from build123d import *

# Parameters (mm, degrees)
SKETCH1_W                   = 20
SKETCH1_H                   = 20
EXTRUDE1_DEPTH              = 10
SKETCH2_R                   = 6
CUT_EXTRUDE1_DEPTH          = 25.494897428
EXTRUDE2_START              = -6
SKETCH4_R                   = 6
SKETCH4_R_2                 = 3.6
EXTRUDE2_DEPTH              = 6
CUT_EXTRUDE5_DEPTH          = 1.4
SKETCH13_R                  = 3.6
EXTRUDE3_DEPTH              = 0.75
SKETCH14_W                  = 6
SKETCH14_H                  = 4.57685066
EXTRUDE4_DEPTH              = 2
EXTRUDE4_DRAFT              = 5
EXTRUDE4_PROFILE_2_DEPTH    = 2
EXTRUDE4_PROFILE_2_DRAFT    = 5
FILLET2_R                   = 2.032
CIRPATTERN1_COUNT           = 2
CIRPATTERN1_ANGLE           = 90
CIRPATTERN1_COPY_1_SKETCH_W = 6
CIRPATTERN1_COPY_1_SKETCH_H = 4.57685066
CIRPATTERN1_COPY_1_DEPTH    = 2
CIRPATTERN1_COPY_1_DRAFT    = 5
CIRPATTERN1_COPY_2_SKETCH_W = 6
CIRPATTERN1_COPY_2_SKETCH_H = 4.57685066
CIRPATTERN1_COPY_2_DEPTH    = 2
CIRPATTERN1_COPY_2_DRAFT    = 5
CIRPATTERN1_COPY_3_SKETCH_W = 6
CIRPATTERN1_COPY_3_SKETCH_H = 4.57685066
CIRPATTERN1_COPY_3_DEPTH    = 2
CIRPATTERN1_COPY_3_DRAFT    = 5
SKETCH12_W                  = 6.3
SKETCH12_H                  = 0.5
CUT_EXTRUDE6_DEPTH          = 26.476901303


with BuildPart() as part:
    # Sketch1 → Extrude1 (new, symmetric)
    with BuildSketch(Plane.XY):
        Rectangle(SKETCH1_W, SKETCH1_H)
    extrude(amount=EXTRUDE1_DEPTH, both=True)

    # Sketch2 → Cut-Extrude1 (cut, through all)
    with BuildSketch(Plane.XY.offset(10)):
        Circle(SKETCH2_R)
    cut_extrude1 = extrude(amount=-CUT_EXTRUDE1_DEPTH, mode=Mode.SUBTRACT)

    # Cut-Extrude2 cone 1 section (through the dimple's axis) → Cut-Extrude2 (revolve, cut)
    with BuildSketch(Plane(origin=(0, 0, 10), x_dir=(0, -1, 0), z_dir=(1, 0, 0))):
        Polygon((0, 0), (7.05, 0), (0, 7.05), align=None)
    cut_extrude2 = revolve(axis=Axis((0, 0, 10), (0, 0, -1)), mode=Mode.SUBTRACT)

    # Sketch4 → Extrude2 (add)
    with BuildSketch(Plane(origin=(0, 0, -10), x_dir=(-1, 0, 0), z_dir=(0, 0, -1)).offset(EXTRUDE2_START)):
        with Locations(Location((0, 0, 0), (0, 0, 180))):
            Circle(SKETCH4_R)
        Circle(SKETCH4_R_2, mode=Mode.SUBTRACT)
    extrude2 = extrude(amount=EXTRUDE2_DEPTH)

    # Sketch10 → Cut-Extrude5 (cut)
    with BuildSketch(Plane(origin=(0, 0, -10), x_dir=(-1, 0, 0), z_dir=(0, 0, -1))):
        Polygon((-5.335281374, 3.15), (-3.15, 5.335281374), (-3.15, 9.5), (3.15, 9.5), (3.15, 5.335281374), (5.335281374, 3.15), (9.5, 3.15), (9.5, -3.15), (5.335281374, -3.15), (3.15, -5.335281374), (3.15, -9.5), (-3.15, -9.5), (-3.15, -5.335281374), (-5.335281374, -3.15), (-9.5, -3.15), (-9.5, 3.15), align=None)
    cut_extrude5 = extrude(amount=-CUT_EXTRUDE5_DEPTH, mode=Mode.SUBTRACT)

    # Sketch13 → Extrude3 (add)
    with BuildSketch(Plane(origin=(0, 0, -8.6), x_dir=(-1, 0, 0), z_dir=(0, 0, -1))):
        Polygon((5.27314934, 3), (5.27314934, -3), (3, -5.27314934), (3, -9.35), (-3, -9.35), (-3, -5.27314934), (-5.27314934, -3), (-5.27314934, 3), (-3, 5.27314934), (-3, 9.35), (3, 9.35), (3, 5.27314934), align=None)
        Circle(SKETCH13_R, mode=Mode.SUBTRACT)
    extrude3 = extrude(amount=EXTRUDE3_DEPTH)


with BuildPart() as extrude4_tool:
    # Sketch14 → Extrude4 (with draft: the straight prism first)
    with BuildSketch(Plane(origin=(0, 0, -9.35), x_dir=(-1, 0, 0), z_dir=(0, 0, -1))):
        with Locations((0, 7.06157467)):
            Rectangle(SKETCH14_W, SKETCH14_H)
    extrude(amount=EXTRUDE4_DEPTH)
    # Extrude4: the draft: its side faces are tilted about the plane it starts from
    extrude4_sides = [extrude4_tool.faces().sort_by_distance(p)[0] for p in [
        (3, 7.06157467, -10.35),
        (0, 4.77314934, -10.35),
        (-3, 7.06157467, -10.35),
        (0, 9.35, -10.35),
    ]]
    draft(extrude4_sides, Plane(origin=(0, 0, -9.35), x_dir=(-1, 0, 0), z_dir=(0, 0, -1)), EXTRUDE4_DRAFT)


with BuildPart() as part_1:
    add(part.part)

    # Extrude4: add extrude4_tool
    add(extrude4_tool.part)


with BuildPart() as extrude4_profile_2_tool:
    # Sketch14 → Extrude4 profile 2 (with draft: the straight prism first)
    with BuildSketch(Plane(origin=(0, 0, -9.35), x_dir=(-1, 0, 0), z_dir=(0, 0, -1))):
        with Locations((0, -7.06157467)):
            Rectangle(SKETCH14_W, SKETCH14_H)
    extrude(amount=EXTRUDE4_PROFILE_2_DEPTH)
    # Extrude4 profile 2: the draft: its side faces are tilted about the plane it starts from
    extrude4_profile_2_sides = [extrude4_profile_2_tool.faces().sort_by_distance(p)[0] for p in [
        (0, -9.35, -10.35),
        (-3, -7.06157467, -10.35),
        (0, -4.77314934, -10.35),
        (3, -7.06157467, -10.35),
    ]]
    draft(extrude4_profile_2_sides, Plane(origin=(0, 0, -9.35), x_dir=(-1, 0, 0), z_dir=(0, 0, -1)), EXTRUDE4_PROFILE_2_DRAFT)


with BuildPart() as part_2:
    add(part_1.part)

    # Extrude4 profile 2: add extrude4_profile_2_tool
    add(extrude4_profile_2_tool.part)

    # Fillet2
    fillet2_edges = [part_2.edges().sort_by_distance(p)[0] for p in [
        (10, 0, 10),
        (-10, 0, 10),
        (0, -10, 10),
        (10, -10, 0),
        (-10, -10, 0),
    ]]
    fillet(fillet2_edges, radius=FILLET2_R)

    # Sketch9 → Revolve1 (revolve)
    with BuildSketch(Plane(origin=(0, 0, 0), x_dir=(0, 0, -1), z_dir=(1, 0, 0)), mode=Mode.PRIVATE) as revolve1_sk:
        with BuildLine():
            Line((-10, 7), (-10, 6))
            Line((-10, 6), (-7, 6))
            Line((-7, 6), (-7, 5.5))
            Line((-7, 5.5), (-10, 5.5))
            Line((-10, 5.5), (-10, 0))
            Line((-10, 0), (-11, 0))
            ThreePointArc((-11, 0), (-10.874840967, 3.508917212), (-10.5, 7))
            Line((-10.5, 7), (-10, 7))
        make_face()
    revolve1 = revolve(revolve1_sk.sketch.rotate(Axis((0, 0, 10), (0, 0, -1)), 180), axis=Axis((0, 0, 10), (0, 0, -1)))

    # CirPattern1: Cut-Extrude1, Cut-Extrude2, Extrude2, Cut-Extrude5, Extrude3, Revolve1 ×2 about axis
    cirpattern1_axis = Axis((0, 0, 0), (1, 0, 0))
    add([cut_extrude1.rotate(cirpattern1_axis, i * CIRPATTERN1_ANGLE / (CIRPATTERN1_COUNT - 1)) for i in range(1, CIRPATTERN1_COUNT)], mode=Mode.SUBTRACT)
    add([cut_extrude2.rotate(cirpattern1_axis, i * CIRPATTERN1_ANGLE / (CIRPATTERN1_COUNT - 1)) for i in range(1, CIRPATTERN1_COUNT)], mode=Mode.SUBTRACT)
    add([extrude2.rotate(cirpattern1_axis, i * CIRPATTERN1_ANGLE / (CIRPATTERN1_COUNT - 1)) for i in range(1, CIRPATTERN1_COUNT)])
    add([cut_extrude5.rotate(cirpattern1_axis, i * CIRPATTERN1_ANGLE / (CIRPATTERN1_COUNT - 1)) for i in range(1, CIRPATTERN1_COUNT)], mode=Mode.SUBTRACT)
    add([extrude3.rotate(cirpattern1_axis, i * CIRPATTERN1_ANGLE / (CIRPATTERN1_COUNT - 1)) for i in range(1, CIRPATTERN1_COUNT)])
    add([revolve1.rotate(cirpattern1_axis, i * CIRPATTERN1_ANGLE / (CIRPATTERN1_COUNT - 1)) for i in range(1, CIRPATTERN1_COUNT)])


with BuildPart() as cirpattern1_copy_1_tool:
    # CirPattern1 copy 1 sketch → CirPattern1 copy 1 (with draft: the straight prism first)
    with BuildSketch(Plane(origin=(0, 9.35, 0), x_dir=(-1, 0, 0), z_dir=(0, 1, 0))):
        with Locations((0, 7.06157467)):
            Rectangle(CIRPATTERN1_COPY_1_SKETCH_W, CIRPATTERN1_COPY_1_SKETCH_H)
    extrude(amount=CIRPATTERN1_COPY_1_DEPTH)
    # CirPattern1 copy 1: the draft: its side faces are tilted about the plane it starts from
    cirpattern1_copy_1_sides = [cirpattern1_copy_1_tool.faces().sort_by_distance(p)[0] for p in [
        (3, 10.35, 7.06157467),
        (0, 10.35, 4.77314934),
        (-3, 10.35, 7.06157467),
        (0, 10.35, 9.35),
    ]]
    draft(cirpattern1_copy_1_sides, Plane(origin=(0, 9.35, 0), x_dir=(-1, 0, 0), z_dir=(0, 1, 0)), CIRPATTERN1_COPY_1_DRAFT)


with BuildPart() as part_3:
    add(part_2.part)

    # CirPattern1 copy 1: add cirpattern1_copy_1_tool
    add(cirpattern1_copy_1_tool.part)


with BuildPart() as cirpattern1_copy_2_tool:
    # CirPattern1 copy 2 sketch → CirPattern1 copy 2 (with draft: the straight prism first)
    with BuildSketch(Plane(origin=(0, 9.35, 0), x_dir=(-1, 0, 0), z_dir=(0, 1, 0))):
        with Locations((0, -7.06157467)):
            Rectangle(CIRPATTERN1_COPY_2_SKETCH_W, CIRPATTERN1_COPY_2_SKETCH_H)
    extrude(amount=CIRPATTERN1_COPY_2_DEPTH)
    # CirPattern1 copy 2: the draft: its side faces are tilted about the plane it starts from
    cirpattern1_copy_2_sides = [cirpattern1_copy_2_tool.faces().sort_by_distance(p)[0] for p in [
        (0, 10.35, -9.35),
        (-3, 10.35, -7.06157467),
        (0, 10.35, -4.77314934),
        (3, 10.35, -7.06157467),
    ]]
    draft(cirpattern1_copy_2_sides, Plane(origin=(0, 9.35, 0), x_dir=(-1, 0, 0), z_dir=(0, 1, 0)), CIRPATTERN1_COPY_2_DRAFT)


with BuildPart() as part_4:
    add(part_3.part)

    # CirPattern1 copy 2: add cirpattern1_copy_2_tool
    add(cirpattern1_copy_2_tool.part)


with BuildPart() as cirpattern1_copy_3_tool:
    # CirPattern1 copy 3 sketch → CirPattern1 copy 3 (with draft: the straight prism first)
    with BuildSketch(Plane(origin=(0, 9.35, 0), x_dir=(-1, 0, 0), z_dir=(0, 1, 0))):
        with Locations((0, -7.06157467)):
            Rectangle(CIRPATTERN1_COPY_3_SKETCH_W, CIRPATTERN1_COPY_3_SKETCH_H)
    extrude(amount=CIRPATTERN1_COPY_3_DEPTH)
    # CirPattern1 copy 3: the draft: its side faces are tilted about the plane it starts from
    cirpattern1_copy_3_sides = [cirpattern1_copy_3_tool.faces().sort_by_distance(p)[0] for p in [
        (0, 10.35, -9.35),
        (-3, 10.35, -7.06157467),
        (0, 10.35, -4.77314934),
        (3, 10.35, -7.06157467),
    ]]
    draft(cirpattern1_copy_3_sides, Plane(origin=(0, 9.35, 0), x_dir=(-1, 0, 0), z_dir=(0, 1, 0)), CIRPATTERN1_COPY_3_DRAFT)


with BuildPart() as part_5:
    add(part_4.part)

    # CirPattern1 copy 3: add cirpattern1_copy_3_tool
    add(cirpattern1_copy_3_tool.part)

    # Sketch12 → Cut-Extrude6 (cut, through all)
    with BuildSketch(Plane.XZ.offset(-9.5)):
        with Locations((0, -9.75)):
            Rectangle(SKETCH12_W, SKETCH12_H)
    extrude(amount=-CUT_EXTRUDE6_DEPTH, mode=Mode.SUBTRACT)


solid = part_5.part
Work out the finished part from the listing and answer in its coordinate system (mm). A direction names the side the tool comes from. Give positions to 0.01 mm unless a question says otherwise; leave off trailing zeros. Answer as a JSON object with one key per item and string values. Group by question number.
1. A tool of negligible diameter and unlimited length cuts with its end or side. For faces 5 (the flat face through (-2, -10, -7)), 6 (the cylindrical face through (-3.434, 6.638, 1.081)), 7 (the flat face through (7, 3.15, -9)), from which of +Z, -Z, +X, -X, +Y, -Y can it reach the whole face along a straight path? Write none if from no direction.
2. Flat-ended cylindrical pins translate along their axes: pin 1 Ø0.7 at (x, y) = (-7.5, 9.5) entering from -Z; pin 2 Ø11 at (x, y) = (-0.5, 0.5) entering from -Z; pin 3 Ø1.5 at (x, z) = (5.5, 6) entering from +Y; pin 4 Ø1.5 at (x, z) = (0.5, 4) entering from -Y. Find the tip coordinate at first contact, or state that the pin passes through.
3. The mould has two halves that part along Y. Classify faces 1 (the flat face through (9.5, 0, -9)), 2 (the flat face through (0, -10, 0)), 3 (the cylindrical face through (0.11, -9.42, 9.39)), 4 (the cylindrical face through (9.42, 1.14, 9.39)): released by +Y, released by -Y, zero draft, split by the parting line, or undercut.
4. Section A-A on x = 6.5 is taken. Count the separate pieces of the cut face and the enclosed holes in it, plus the area to 3 significant figures.
5. Consider line 1 along Y through (x, z) = (-3.75, 9.75); line 2 along X through (y, z) = (0, -6.2); line 3 along Z through (x, y) = (-1.25, 5.5). Determine where each line is inside the solid, lowest interval first. Write a range as [from, to].
Result sheet:
{
 "1": {"face 5": "-Y", "face 6": "+Y", "face 7": "-Z"},
 "2": {"pin 1": "stops at z = -10", "pin 2": "stops at z = -11.35", "pin 3": "stops at y = 10", "pin 4": "stops at y = -10.89"},
 "3": {"face 1": "undercut", "face 2": "undercut", "face 3": "released by -Y", "face 4": "zero draft"},
 "4": {"separate pieces": "3", "enclosed holes": "0", "area": "383 mm^2"},
 "5": {"line 1": "y = [-8.94, -5.67], [-4.68, -4.02], [4.02, 4.68], [5.67, 10]", "line 2": "x = [-10, -3.6], [3.6, 10]", "line 3": "z = [-11.35, -3.38], [3.38, 5.87], [7, 10.68]"}
}
